Work out the finished part from the listing and answer in its coordinate system (mm). A direction names the side the tool comes from. Coordinates: 2 decimals unless noted, no trailing zeros. Write each loop counter-clockwise with the first axis right and the second up, starting at its lowest first coordinate (ties: lowest second). Pieces come first, ordered by that corner, then holes. Notation, with made-up numbers: (86, 63) - (118, 63) arc R14 cw to (118, 75) - close; hole circle Ø2 at (65, 3). An arc over 180 degrees is marked (long way). Use a Markdown table: item, result. Add a question column.
(1) Find the intervals of material crossed by line 1 (Z direction, x = -111, y = 52); line 2 (Y direction, x = -89, z = 10); line 3 (X direction, y = 49.75, z = 14), in increasing order. Write a range as from..to.
(2) For a pull along Y with two mould halves and no side action, classify faces 3 (the face through (-101.034, 50.226, 9.077)), 4 (the face through (-121, 51, 12)), 5 (the face through (-112.323, 48.095, 10.867)) as released by +Y, released by -Y, zero draft, split by the parting line, or undercut.
(3) Given pin 1 Ø2 at (x, y) = (-98.5, 50.5) entering from +Z; pin 2 Ø3.5 at (y, z) = (52, 10) entering from -X; pin 3 Ø1.5 at (x, y) = (-113.5, 51) entering from -Z; pin 4 Ø2 at (x, y) = (-115.5, 48.5) entering from +Z, each flat-ended and moving along its own axis, determine where each tip first touches the part or whether it passes through.
(4) The part is cut by section B-B, the plane z = 10. Give the vertices of the cut face in (x, y).
(5) The part is cut by section D-D, the plane y = 54.5. Give the vertices of the cut face in (x, z).
(6) A tool of negligible diameter and unlimited length cuts with its end or side. For faces 1 (the face through (-80.5, 51, 12)), 2 (the face through (-91.4, 48.095, 10.867)), from which of +Z, -Z, +X, -X, +Y, -Y can it reach the whole face along a straight path? Write none if from no direction.
(7) The part is cut by section A-A, the plane y = 52. Give the vertices of the cut face in (x, z).
(8) The part is cut by section C-C, the plane x = -103. Give the vertices of the cut face in (y, z).
from build123d import *

# Parameters (mm, degrees)
CYLINDER138_R     = 2
CYLINDER138_DEPTH = 47.8
CYLINDER091_R     = 5
CYLINDER091_DEPTH = 1.4
CYLINDER072_R     = 4
CYLINDER072_DEPTH = 40.5


with BuildPart() as cylinder138:
    # Cylinder138 → Cylinder138 (new body)
    with BuildSketch(Plane(origin=(-125, 62, 10), x_dir=(0, 0, -1), z_dir=(1, 0, 0))):
        Circle(CYLINDER138_R)
    extrude(amount=CYLINDER138_DEPTH)


with BuildPart() as cylinder091:
    # Cylinder091 → Cylinder091 (new body)
    with BuildSketch(Plane(origin=(-107.4, 62, 10), x_dir=(0, 0, -1), z_dir=(1, 0, 0))):
        Circle(CYLINDER091_R)
    extrude(amount=CYLINDER091_DEPTH)


with BuildPart() as cut095:
    # Cylinder072 → Cylinder072 (new body)
    with BuildSketch(Plane(origin=(-125, 62, 10), x_dir=(0, 0, -1), z_dir=(1, 0, 0))):
        Circle(CYLINDER072_R)
    extrude(amount=CYLINDER072_DEPTH)

    # Fusion142: union Cylinder091
    add(cylinder091.part)

    # Cut095: cut Cylinder138
    add(cylinder138.part, mode=Mode.SUBTRACT)


with BuildPart() as cut095_1:
    # Cut095 placement: moved
    add(cut095.part.moved(Location((4, -10, 0))))


solid = cut095_1.part
Model answer:
| question | item | result |
|---|---|---|
| 1 | line 1 | 6..8, 12..14 |
| 1 | line 2 | 48..50, 54..56 |
| 1 | line 3 | -103.4..-102 |
| 2 | face 3 | undercut |
| 2 | face 4 | zero draft |
| 2 | face 5 | split by the parting line |
| 3 | pin 1 | z = 13.97 |
| 3 | pin 2 | through |
| 3 | pin 3 | z = 6.01 |
| 3 | pin 4 | z = 13.12 |
| 4 | outline | (-121, 48) - (-103.4, 48) - (-103.4, 47) - (-102, 47) - (-102, 48) - (-80.5, 48) - (-80.5, 50) - (-121, 50) - close; (-121, 54) - (-80.5, 54) - (-80.5, 56) - (-102, 56) - (-102, 57) - (-103.4, 57) - (-103.4, 56) - (-121, 56) - close |
| 5 | outline | (-121, 6.88) - (-103.4, 6.88) - (-103.4, 5.67) - (-102, 5.67) - (-102, 6.88) - (-80.5, 6.88) - (-80.5, 13.12) - (-102, 13.12) - (-102, 14.33) - (-103.4, 14.33) - (-103.4, 13.12) - (-121, 13.12) - close |
| 6 | face 1 | +Z, -Z, +X, +Y, -Y |
| 6 | face 2 | +X |
| 7 | outline | (-121, 6) - (-103.4, 6) - (-103.4, 5) - (-102, 5) - (-102, 6) - (-80.5, 6) - (-80.5, 8) - (-121, 8) - close; (-121, 12) - (-80.5, 12) - (-80.5, 14) - (-102, 14) - (-102, 15) - (-103.4, 15) - (-103.4, 14) - (-121, 14) - close |
| 8 | outline | circle Ø10 at (52, 10); hole circle Ø4 at (52, 10) |
